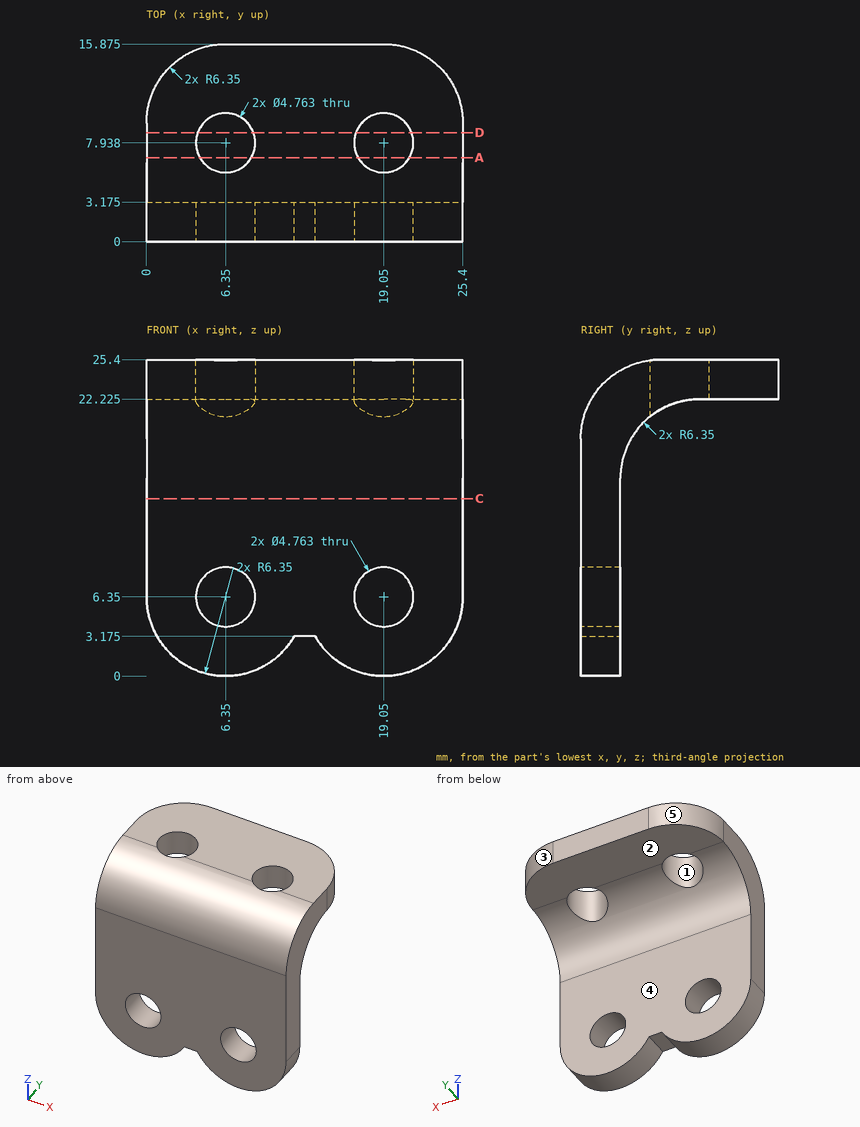
Here's the drawing with two shaded views (mm, measured from the low corner). I have some questions. A direction names the side the tool comes from. Round coordinates to 2 decimals unless told otherwise and drop trailing zeros. Loops run counter-clockwise (first coordinate to the right, second up) from the corner with the lowest first, then second, coordinate; pieces in that order, holes last.
Item 1: Suppose I cut it at C-C, the plane z = 14.25. Write out the boundary of the cut face in (x, y) (1 decimal).
Item 2: Will these pins go through, and if not, where does the flat tip stop? pin 1 Ø4.5 at (x, z) = (19.05, 6.35) entering from -Y; pin 2 Ø0.9 at (x, y) = (12.5, 2) entering from -Z (1 decimal); pin 3 Ø8 at (x, z) = (9.5, 7.5) entering from +Y (1 decimal); pin 4 Ø5 at (x, y) = (9.5, 14) entering from -Z (1 decimal).
Item 3: Suppose I cut it at A-A, the plane y = 6.75. Write out the boundary of the cut face in (x, z) (1 decimal).
Item 4: Which directions (+Z, -Z, +X, -X, +Y, -Y) give clear straight access to the entire face, cutting with the end or side of a thin tool? Please do the marked faces 4 and 5.
Item 5: Suppose I cut it at D-D, the plane y = 8.75. Write out the boundary of the cut face in (x, z).
Item 6: Please list where these lines run through material, in increasing order: L1, parallel to X at y = 2.5, z = 8 (1 decimal); L2, parallel to Z at x = 22.25, y = 14.75 (1 decimal); L3, parallel to Y at x = 21.75, z = 11.75 (1 decimal).
Item 7: If we mould it in two halves opening along X, with no side actions, what happens to the marked faces 1, 2 and 3? For each: +X half, -X half, draft (parallel to the pull), parting line (faces both ways), or undercut.
Reported:
1. outline: (0, 0) - (25.4, 0) - (25.4, 3.2) - (0, 3.2) - close
2. pin 1: passes through
2. pin 2: stops at z = 3.2
2. pin 3: stops at y = 3.2
2. pin 4: stops at z = 22.2
3. outline: (0, 21.6) - (4.3, 21.6) - (4.3, 25.4) - (0, 25.4) - close; (8.4, 21.6) - (17, 21.6) - (17, 25.4) - (8.4, 25.4) - close; (21.1, 21.6) - (25.4, 21.6) - (25.4, 25.4) - (21.1, 25.4) - close
4. face 4: -Z, +X, -X, +Y
4. face 5: +Z, -Z, -X, +Y
5. outline: (0, 22.18) - (4.11, 22.18) - (4.11, 25.4) - (0, 25.4) - close; (8.59, 22.18) - (16.81, 22.18) - (16.81, 25.4) - (8.59, 25.4) - close; (21.29, 22.18) - (25.4, 22.18) - (25.4, 25.4) - (21.29, 25.4) - close
6. L1: x = 0 to 4.6, 8.1 to 17.3, 20.8 to 25.4
6. L2: z = 22.2 to 25.4
6. L3: y = 0 to 3.2
7. face 1: undercut
7. face 2: draft
7. face 3: +X half
